from build123d import *

# Parameters (mm, degrees)
F0_R     = 13.5
F0_R_2   = 9.3155
F1_DEPTH = 11
F2_R     = 13.5
F2_R_2   = 12
F3_DEPTH = 32
F4_R     = 13.5
F4_R_2   = 9.3155
F5_DEPTH = 11
F6_R     = 13.5
F6_R_2   = 12
F7_DEPTH = 16
F8_R     = 13.5
F8_R_2   = 9.3155
F9_DEPTH = 11


with BuildPart() as f1:
    # F0 (on Front) → F1 (new body)
    with BuildSketch(Plane.XZ):
        Circle(F0_R)
        Circle(F0_R_2, mode=Mode.SUBTRACT)
    extrude(amount=F1_DEPTH)

    # F2 (on face) → F3 (join)
    with BuildSketch(Plane(origin=(0, 0, 0), x_dir=(-1, 0, 0), z_dir=(0, 1, 0))):
        Circle(F2_R)
        Circle(F2_R_2, mode=Mode.SUBTRACT)
    extrude(amount=F3_DEPTH)

    # F4 (on face) → F5 (join)
    with BuildSketch(Plane(origin=(0, 32, 0), x_dir=(-1, 0, 0), z_dir=(0, 1, 0))):
        Circle(F4_R)
        Circle(F4_R_2, mode=Mode.SUBTRACT)
    extrude(amount=F5_DEPTH)

    # F6 (on Top) → F7 (join)
    with BuildSketch(Plane.XY):
        with Locations((0, 16)):
            Circle(F6_R)
        with Locations((0, 16)):
            Circle(F6_R_2, mode=Mode.SUBTRACT)
    extrude(amount=F7_DEPTH)

    # F8 (on face) → F9 (join)
    with BuildSketch(Plane.XY.offset(16)):
        with Locations((0, 16)):
            Circle(F8_R)
        with Locations((0, 16)):
            Circle(F8_R_2, mode=Mode.SUBTRACT)
    extrude(amount=F9_DEPTH)


solid = f1.part
Design review of the part built by this model. Coordinates are the model's own, in mm. A direction names the side the tool comes from. Round coordinates to 2 decimals unless told otherwise and drop trailing zeros. Write each loop counter-clockwise with the first axis right and the second up, starting at its lowest first coordinate (ties: lowest second). Pieces come first, ordered by that corner, then holes.
Item 1: Consider section C-C on y = -2. Give the boundary of the cut face in (x, z), and give its area (3 significant figures).
Item 2: Draft analysis for pull direction Z (two halves, no side actions). For faces 5 (the cylindrical face through (-8.885, 37.423, 2.798)), 6 (the flat face through (9, 19, 27)), 7 (the cylindrical face through (0, 4, 5)), 8 (the flat face through (-9, 43, 3)), state which applies: released by +Z, released by -Z, zero draft, split by the parting line, or undercut.
Item 3: Wall thickness on L1, parallel to Y at x = 0, z = 11.5; L2, parallel to Y at x = 8.5, z = -7; L3, parallel to Y at x = 1.25, z = 10: over which ranges is each line inside the solid? List them lowest first.
Item 4: For pin 1 Ø15 at (x, z) = (0, 0) entering from -Y; pin 2 Ø2 at (y, z) = (33.5, 5) entering from +X; pin 3 Ø2 at (x, y) = (-5.5, 22) entering from +Z, all flat-tipped, find the tip position at first contact; note any pin that passes through.
Item 5: Consider section B-B on z = 5. Give the boundary of the cut face in (x, y).
Item 6: Consider section A-A on y = 6. Give the boundary of the cut face in (x, z), and give its area (3 significant figures).
Item 7: For faces 1 (the flat face through (9, -11, 3)), 2 (the cylindrical face through (8.885, -5.423, 2.798)), 3 (the cylindrical face through (-2, 6.9, 21.4)), 4 (the cylindrical face through (2.601, 15.776, -11.715)), list the 3-axis set-ups (+Z, -Z, +X, -X, +Y, -Y) from which the entire face can be reached by the end or side of a thin tool; tool diameter is ignored.
Item 8: Consider section D-D on x = -11. Give the boundary of the cut face in (y, z), and give its area (3 significant figures).
Check values:
1. outline: circle Ø27 at (0, 0); hole circle Ø18.63 at (0, 0)
1. area: 300 mm2
2. face 5: undercut
2. face 6: released by +Z
2. face 7: undercut
2. face 8: zero draft
3. L1: y = -11 to 0, 2.5 to 4, 28 to 29.5, 32 to 43
3. L2: y = -11 to 0, 32 to 43
3. L3: y = -11 to 0, 2.56 to 4.07, 27.93 to 29.44, 32 to 43
4. pin 1: stops at y = 2.5
4. pin 2: stops at x = 12.89
4. pin 3: stops at z = 12.73
5. outline: (-12.54, -11) - (-7.86, -11) - (-7.86, 0) - (-10.91, 0) - (-10.91, 8.05) arc R13.5 ccw to (10.91, 8.05) - (10.91, 0) - (7.86, 0) - (7.86, -11) - (12.54, -11) - (12.54, 11) arc R13.5 ccw to (12.54, 21) - (12.54, 43) - (7.86, 43) - (7.86, 32) - (10.91, 32) - (10.91, 23.95) arc R13.5 ccw to (-10.91, 23.95) - (-10.91, 32) - (-7.86, 32) - (-7.86, 43) - (-12.54, 43) - (-12.54, 21) arc R13.5 ccw to (-12.54, 11) - close; hole (-10.91, 11) arc R12 ccw to (10.91, 11) - (10.91, 21) arc R12 ccw to (-10.91, 21) - close
6. outline: (-9.07, 10) arc R13.5 ccw (long way) to (9.07, 10) - (9.07, 27) - (-9.07, 27) - close; hole (-9.07, 0) - (-9.07, 7.86) arc R12 ccw (long way) to (9.07, 7.86) - (9.07, 0) - (6.63, 0) - (6.63, 10) arc R12 ccw to (-6.63, 10) - (-6.63, 0) - close; hole (-6.63, 11.76) arc R13.5 cw to (6.63, 11.76) - (6.63, 16) - (-6.63, 16) - close
6. area: 388 mm2
7. face 1: +Z, -Z, +X, -X, -Y
7. face 2: -Y
7. face 3: +Z
7. face 4: none
8. outline: (-11, -7.83) - (43, -7.83) - (43, 7.83) - (23.83, 7.83) - (23.83, 27) - (8.17, 27) - (8.17, 7.83) - (-11, 7.83) - close; hole (0, -4.8) - (32, -4.8) - (32, 4.8) - (23.83, 4.8) - (23.83, 0) - (20.8, 0) - (20.8, 4.8) - (11.2, 4.8) - (11.2, 0) - (8.17, 0) - (8.17, 4.8) - (0, 4.8) - close; hole (11.2, 7.83) - (20.8, 7.83) - (20.8, 16) - (11.2, 16) - close
8. area: 789 mm2
